from build123d import *

# Parameters (mm, degrees)
SKETCH_1_R          = 4.2
EXTRUDE_1_DEPTH     = 4.84
SKETCH_2_R          = 2.5
EXTRUDE_2_DEPTH     = 25
CUT_EXTRUDE_1_DEPTH = 3.4


with BuildPart() as part:
    # 草图1 → 凸台-拉伸1 (new body)
    with BuildSketch(Plane(origin=(0, 0, 0), x_dir=(1, 0, 0), z_dir=(0, 1, 0))):
        Circle(SKETCH_1_R)
    extrude(amount=EXTRUDE_1_DEPTH)

    # 草图2 → 凸台-拉伸2 (add)
    with BuildSketch(Plane(origin=(0, 4.84, 0), x_dir=(1, 0, 0), z_dir=(0, 1, 0))):
        Circle(SKETCH_2_R)
    extrude(amount=EXTRUDE_2_DEPTH)

    # 草图3 → 切除-拉伸1 (cut)
    with BuildSketch(Plane.XZ):
        Polygon((2.3, 0), (1.15, 1.991858429), (-1.15, 1.991858429), (-2.3, 0), (-1.15, -1.991858429), (1.15, -1.991858429), align=None)
    extrude(amount=-CUT_EXTRUDE_1_DEPTH, mode=Mode.SUBTRACT)


solid = part.part
Read the model definition and answer for the solid it produces. Units are mm, in the model's axes. A direction names the side the tool comes from. Coordinates: 2 decimals unless noted, no trailing zeros. Write each loop counter-clockwise with the first axis right and the second up, starting at its lowest first coordinate (ties: lowest second). Pieces come first, ordered by that corner, then holes. Notation, with made-up numbers: M -15,14.5 L 19,14.5 A12 ccw 19,22.5 Z; hole C 35.25,-9.75 d6. An arc over 180 degrees is marked long. Use a Markdown table: item, result.
Q1. Each of these flat-tipped pins is pushed along its axis until it touches: pin 1 Ø4.5 at (x, z) = (0, 0) entering from -Y; pin 2 Ø4 at (x, y) = (-2.5, 18.5) entering from -Z; pin 3 Ø1.5 at (y, z) = (25, 2.5) entering from -X; pin 4 Ø4 at (x, y) = (3, 19.5) entering from -Z. Where does it stop, or does it pass through?
Answer block:
| item | result |
|---|---|
| pin 1 | stops at y = 0 |
| pin 2 | stops at z = -2.45 |
| pin 3 | stops at x = -1.79 |
| pin 4 | stops at z = -2.29 |
Q2. The part is cut by section C-C, the plane y = 5.25. Write down the section's boundary in (x, z).
Answer block:
| item | result |
|---|---|
| outline | C 0,0 d5 |
Q3. Straight lines are drawn through the part: L1, parallel to Y at x = 1, z = 2.75; L2, parallel to Y at x = -1, z = -1.75; L3, parallel to X at y = 3.25, z = 0.25. For each, find the intervals that lie inside material, in ascending order. Write a range as [from, to].
Answer block:
| item | result |
|---|---|
| L1 | y = [0, 4.84] |
| L2 | y = [3.4, 29.84] |
| L3 | x = [-4.19, -2.16], [2.16, 4.19] |
Q4. The part is cut by section D-D, the plane z = 3. Write down the section's boundary in (x, y).
Answer block:
| item | result |
|---|---|
| outline | M -2.94,0 L 2.94,0 L 2.94,4.84 L -2.94,4.84 Z |
Q5. The part is cut by section B-B, the plane z = 1.5. Write down the section's boundary in (x, y).
Answer block:
| item | result |
|---|---|
| outline | M -3.92,0 L -1.43,0 L -1.43,3.4 L 1.43,3.4 L 1.43,0 L 3.92,0 L 3.92,4.84 L 2,4.84 L 2,29.84 L -2,29.84 L -2,4.84 L -3.92,4.84 Z |
Q6. The part is cut by section A-A, the plane x = 0. Write down the section's boundary in (y, z), then the cut area to 3 significant figures.
Answer block:
| item | result |
|---|---|
| outline | M 0,-4.2 L 4.84,-4.2 L 4.84,-2.5 L 29.84,-2.5 L 29.84,2.5 L 4.84,2.5 L 4.84,4.2 L 0,4.2 L 0,1.99 L 3.4,1.99 L 3.4,-1.99 L 0,-1.99 Z |
| area | 152 mm2 |
Q7. Which of the six approach directions +Z, -Z, +X, -X, +Y, -Y give full straight-line access (tool end or side, diameter ignored) to faces 1 (the face through (2, 0, 1)), 2 (the face through (1.733, 1.676, 0.982)), 3 (the face through (-0.54, 17.16, 2.44))?
Answer block:
| item | result |
|---|---|
| face 1 | +Z, -Z, +X, -X, -Y |
| face 2 | -Y |
| face 3 | +Y |
Q8. Determine the mould class of faces 4 (the face through (4.006, 2.386, -1.262)), 5 (the face through (1.717, 1.676, -1.01)), 6 (the face through (2, 4.84, 2)) for opening direction X: released by +X, released by -X, zero draft, split by the parting line, or undercut.
Answer block:
| item | result |
|---|---|
| face 4 | split by the parting line |
| face 5 | undercut |
| face 6 | zero draft |
